The model under review builds one solid part; all positions refer to its coordinate system, in mm. Face numbers are marked on the shaded views. A direction names the side the tool comes from. Coordinates: 2 decimals unless noted, no trailing zeros. Write each loop counter-clockwise with the first axis right and the second up, starting at its lowest first coordinate (ties: lowest second). Pieces come first, ordered by that corner, then holes. Notation, with made-up numbers: (-8, -5) - (35, -5) arc R33 ccw to (35, 24) - close; hole circle Ø8 at (32.5, 62). An arc over 180 degrees is marked (long way). Return JSON: item names as keys, results as strings. Group by question number.
(1) We need section D-D on z = 35. State the section outline as (x, y) points, then the cut area to 3 significant figures.
(2) We need section B-B on y = 0. State the section outline as (x, z) points.
(3) We need section C-C on y = 22.5. State the section outline as (x, z) points.
(4) Tool access review of the marked faces 1 and 2: name each direction out of +Z, -Z, +X, -X, +Y, -Y from which nothing blocks a thin tool from reaching the whole face with its end or side.
(5) We need section A-A on x = 0. State the section outline as (y, z) points.
(6) To check wall thickness, follow L1, parallel to Y at x = 0, z = 3; L2, parallel to Z at x = -27, y = -6; L3, parallel to Y at x = 0, z = 6. State the ranges of each line that lie inside material, in increasing order. Write a range as from..to.
(7) For pin 1 Ø9 at (x, y) = (19.49, 11.25) entering from +Z; pin 2 Ø3.5 at (x, y) = (0, 22.5) entering from +Z; pin 3 Ø8 at (y, z) = (-3, 27) entering from +X; pin 4 Ø5 at (y, z) = (10.5, 12.5) entering from +X, all flat-tipped, find the tip position at first contact; note any pin that passes through.
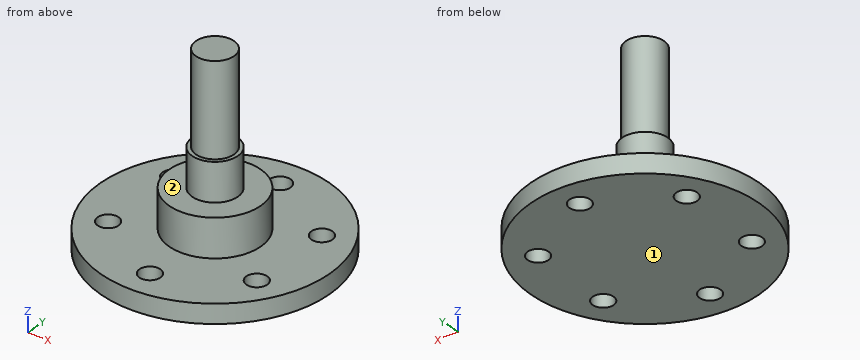
```python
from build123d import *

# Parameters (mm, degrees)
SKETCH_1_R      = 30
SKETCH_1_R_2    = 2.75
EXTRUDE_1_DEPTH = 5
SKETCH_2_R      = 12
EXTRUDE_2_DEPTH = 10
SKETCH_3_R      = 6
EXTRUDE_3_DEPTH = 10
SKETCH_5_R      = 5
EXTRUDE_4_DEPTH = 24.1


with BuildPart() as part:
    # 草图1 → 凸台-拉伸1 (new body)
    with BuildSketch(Plane.XY):
        Circle(SKETCH_1_R)
        with Locations((0, 22.5)):
            Circle(SKETCH_1_R_2, mode=Mode.SUBTRACT)
        with Locations((19.485571585, 11.25)):
            Circle(SKETCH_1_R_2, mode=Mode.SUBTRACT)
        with Locations((19.485571585, -11.25)):
            Circle(SKETCH_1_R_2, mode=Mode.SUBTRACT)
        with Locations((0, -22.5)):
            Circle(SKETCH_1_R_2, mode=Mode.SUBTRACT)
        with Locations((-19.485571585, -11.25)):
            Circle(SKETCH_1_R_2, mode=Mode.SUBTRACT)
        with Locations((-19.485571585, 11.25)):
            Circle(SKETCH_1_R_2, mode=Mode.SUBTRACT)
    extrude(amount=EXTRUDE_1_DEPTH)

    # 草图2 → 凸台-拉伸2 (add)
    with BuildSketch(Plane.XY.offset(5)):
        Circle(SKETCH_2_R)
    extrude(amount=EXTRUDE_2_DEPTH)

    # 草图3 → 凸台-拉伸3 (add)
    with BuildSketch(Plane.XY.offset(15)):
        Circle(SKETCH_3_R)
    extrude(amount=EXTRUDE_3_DEPTH)

    # 草图5 → 凸台-拉伸4 (add)
    with BuildSketch(Plane.XY.offset(25)):
        Circle(SKETCH_5_R)
    extrude(amount=EXTRUDE_4_DEPTH)


solid = part.part
```
Ans:
{
 "1": {"outline": "circle Ø10 at (0, 0)", "area": "78.5 mm²"},
 "2": {"outline": "(-30, 0) - (30, 0) - (30, 5) - (12, 5) - (12, 15) - (6, 15) - (6, 25) - (5, 25) - (5, 49.1) - (-5, 49.1) - (-5, 25) - (-6, 25) - (-6, 15) - (-12, 15) - (-12, 5) - (-30, 5) - close"},
 "3": {"outline": "(-19.84, 0) - (-2.75, 0) - (-2.75, 5) - (-19.84, 5) - close; (2.75, 0) - (19.84, 0) - (19.84, 5) - (2.75, 5) - close"},
 "4": {"face 1": "-Z, +X, -X, +Y, -Y", "face 2": "+Z"},
 "5": {"outline": "(-30, 0) - (-25.25, 0) - (-25.25, 5) - (-30, 5) - close; (-19.75, 0) - (19.75, 0) - (19.75, 5) - (12, 5) - (12, 15) - (6, 15) - (6, 25) - (5, 25) - (5, 49.1) - (-5, 49.1) - (-5, 25) - (-6, 25) - (-6, 15) - (-12, 15) - (-12, 5) - (-19.75, 5) - close; (25.25, 0) - (30, 0) - (30, 5) - (25.25, 5) - close"},
 "6": {"L1": "-30..-25.25, -19.75..19.75, 25.25..30", "L2": "0..5", "L3": "-12..12"},
 "7": {"pin 1": "z = 5", "pin 2": "through", "pin 3": "x = 6", "pin 4": "x = 8.94"}
}
